```python
from build123d import *

# Parameters (mm, degrees)
F1_DEPTH = 24
F3_DEPTH = 11
F5_R     = 13
F6_R     = 5
F4_R     = 2.5
F4_R_2   = 5
F7_DEPTH = 38.1


with BuildPart() as f1:
    # F0 (on Front) → F1 (new body, symmetric)
    with BuildSketch(Plane.XZ):
        with BuildLine():
            Line((19, 0), (51, 0))
            Line((51, 0), (51, 41))
            Line((51, 41), (40, 41))
            Line((40, 41), (40, 11))
            Line((40, 11), (27.910571, 11))
            ThreePointArc((27.910571, 11), (0, 30), (-27.910571, 11))
            Line((-27.910571, 11), (-56, 11))
            Line((-56, 11), (-56, 0))
            Line((-56, 0), (-19, 0))
            ThreePointArc((-19, 0), (0, 19), (19, 0))
        make_face()
    extrude(amount=F1_DEPTH, both=True)

    # F2 (on face) → F3 (cut, through all)
    with BuildSketch(Plane.YZ.offset(51)):
        with BuildLine():
            ThreePointArc((6.5, 25), (0, 31.5), (-6.5, 25))
            ThreePointArc((-6.5, 25), (0, 18.5), (6.5, 25))
        make_face()
        with BuildLine():
            Line((6.5, 41), (-6.5, 41))
            Line((-6.5, 41), (-6.5, 25))
            ThreePointArc((-6.5, 25), (0, 31.5), (6.5, 25))
            Line((6.5, 25), (6.5, 41))
        make_face()
    extrude(amount=-F3_DEPTH, mode=Mode.SUBTRACT)

    # F5
    f5_edges = [f1.edges().sort_by_distance(p)[0] for p in [
        (-56, -24, 5.5),
        (-56, 24, 5.5),
    ]]
    fillet(f5_edges, radius=F5_R)

    # F6
    f6_edges = [f1.edges().sort_by_distance(p)[0] for p in [
        (45.5, -24, 41),
        (45.5, 24, 41),
    ]]
    fillet(f6_edges, radius=F6_R)

    # F4 (on face) → F7 (cut, symmetric)
    with BuildSketch(Plane.XY.offset(11)):
        Circle(F4_R)
        with Locations((-43, -11)):
            Circle(F4_R_2)
        with Locations((-43, 11)):
            Circle(F4_R_2)
    extrude(amount=F7_DEPTH, both=True, mode=Mode.SUBTRACT)


solid = f1.part
```
Part model, mm, in its own coordinate system. A direction names the side the tool comes from. Round coordinates to 2 decimals unless told otherwise and drop trailing zeros. Order: outer loops, then holes, each group sorted by start corner. A loop starts at its lowest first (then second) coordinate and runs counter-clockwise, first axis right, second up. Notation, with made-up numbers: M 12,-28.75 L 65,-28.75 A13 ccw 65,-5.75 Z; hole C -17.75,33 d7. An arc over 180 degrees is marked long. Answer in a Markdown table with one row per item. Add a question column.
Q1. Cut at D-D on y = 15. Give the cut face in (x, z).
Q2. Pin check, flat tips, straight feed: pin 1 (6 mm diameter, centred on y = 8.5, z = 35, fed in from -X); pin 2 (8 mm diameter, centred on x = 0, y = 0, fed in from +Z); pin 3 (9 mm diameter, centred on y = -0.5, z = 19.5, fed in from -X). Stop position of each tip, or through.
Q3. Mould opens along X. For faces 4 (the face through (-52.091, 20.293, 5.423)), 5 (the face through (34, 0, 11)), 6 (the face through (46, -13, 41)) say: +X half, -X half, draft (parallel to the pull), parting line (faces both ways), or undercut.
Q4. Cut at C-C on z = 31. Give the cut face in (x, y), and give its area (3 significant figures).
Q5. 3-axis set-ups, long thin cutter, end or side, ignore diameter. For faces 1 (the face through (45, 23, 39)), 2 (the face through (40, -6, 20)), 3 (the face through (46, 6.5, 33)): which of +Z, -Z, +X, -X, +Y, -Y reach the whole face in a straight line?
Q6. Cut at B-B on z = 5.5. Give the cut face in (x, y).
Q7. Wall check: L1, parallel to Y at x = -43, z = 3.25; L2, parallel to Y at x = 0, z = 22; L3, parallel to X at y = 2.5, z = 13. Give the ranges that are in metal, low to high. Write a range as from..to.
Q8. Cut at A-A on x = 0. Give the cut face in (y, z), and give its area (3 significant figures).
Established:
| question | item | result |
|---|---|---|
| 1 | outline | M -55.37,0 L -46,0 L -46,11 L -55.37,11 Z; M -40,0 L -19,0 A19 cw 19,0 L 51,0 L 51,41 L 40,41 L 40,11 L 27.91,11 A30 ccw -27.91,11 L -40,11 Z |
| 2 | pin 1 | stops at x = 40 |
| 2 | pin 2 | stops at z = 30 |
| 2 | pin 3 | stops at x = -25.98 |
| 3 | face 4 | -X half |
| 3 | face 5 | undercut |
| 3 | face 6 | draft |
| 4 | outline | M 40,-24 L 51,-24 L 51,-6.5 L 40,-6.5 Z; M 40,6.5 L 51,6.5 L 51,24 L 40,24 Z |
| 4 | area | 385 mm2 |
| 5 | face 1 | +Z, +X, -X, +Y |
| 5 | face 2 | +Z, +Y, -Y |
| 5 | face 3 | +Z, +X |
| 6 | outline | M -56,-11 A13 ccw -43,-24 L -18.19,-24 L -18.19,24 L -43,24 A13 ccw -56,11 Z; M 18.19,-24 L 51,-24 L 51,24 L 18.19,24 Z; hole C -43,-11 d10; hole C -43,11 d10 |
| 7 | L1 | y = -24..-16, -6..6, 16..24 |
| 7 | L2 | y = -24..-2.5, 2.5..24 |
| 7 | L3 | x = -27.04..-13.86, 13.86..27.04, 40..51 |
| 8 | outline | M -24,19 L -2.5,19 L -2.5,30 L -24,30 Z; M 2.5,19 L 24,19 L 24,30 L 2.5,30 Z |
| 8 | area | 473 mm2 |
